```python
from build123d import *

# Parameters (mm, degrees)
F1_DEPTH  = 27
F2_R      = 4
F3_DEPTH  = 2
F4_DEPTH  = 29
F5_R      = 9.5
F6_DEPTH  = 4.5
F7_DEPTH  = 31.5
F8_R      = 4
F9_DEPTH  = 1
F11_DEPTH = 15
F12_R     = 4
F13_DEPTH = 0.1
F14_R     = 18.5
F15_DEPTH = 58
F16_R     = 2
F17_DEPTH = 1.5
F18_R     = 1.49999
F19_R     = 2
F20_DEPTH = 5
F21_R     = 2
F22_DEPTH = 5


# Not quite as in the source:
# - a fillet or chamfer is up to 0.001 mm smaller than in the source, because OpenCascade refuses the exact size


with BuildPart() as f1:
    # F0 (on Top) → F1 (new body)
    with BuildSketch(Plane.XY):
        with BuildLine():
            ThreePointArc((38, 17), (37.1213203436, 19.1213203436), (35, 20))
            Line((35, 20), (-17, 20))
            ThreePointArc((-17, 20), (-19.1213203436, 19.1213203436), (-20, 17))
            Line((-20, 17), (-20, -17))
            ThreePointArc((-20, -17), (-19.1213203436, -19.1213203436), (-17, -20))
            Line((-17, -20), (35, -20))
            ThreePointArc((35, -20), (37.1213203436, -19.1213203436), (38, -17))
            Line((38, -17), (38, 17))
        make_face()
    extrude(amount=F1_DEPTH)

    # F2 (on face) → F3 (join)
    with BuildSketch(Plane.XY.offset(27)):
        with Locations((-11, 14)):
            Circle(F2_R)
        with Locations((29, 14)):
            Circle(F2_R)
        with Locations((-11, -14)):
            Circle(F2_R)
        with BuildLine():
            Line((32.4641016151, -12), (29.9641016151, -7.6698729811))
            ThreePointArc((29.9641016151, -7.6698729811), (24.5, -6.2057713659), (23.0358983849, -11.6698729811))
            Line((23.0358983849, -11.6698729811), (25.5358983849, -16))
            ThreePointArc((25.5358983849, -16), (31, -17.4641016151), (32.4641016151, -12))
        make_face()
        with Locations((15.5, 6)):
            Circle(F2_R)
        with Locations((15.5, -6)):
            Circle(F2_R)
    extrude(amount=F3_DEPTH)

    # F2 (on face) → F4 (join)
    with BuildSketch(Plane.XY.offset(27)):
        with Locations((-11, 14)):
            Circle(F2_R)
        with Locations((29, 14)):
            Circle(F2_R)
        with Locations((-11, -14)):
            Circle(F2_R)
        with BuildLine():
            Line((32.4641016151, -12), (29.9641016151, -7.6698729811))
            ThreePointArc((29.9641016151, -7.6698729811), (24.5, -6.2057713659), (23.0358983849, -11.6698729811))
            Line((23.0358983849, -11.6698729811), (25.5358983849, -16))
            ThreePointArc((25.5358983849, -16), (31, -17.4641016151), (32.4641016151, -12))
        make_face()
        with Locations((15.5, 6)):
            Circle(F2_R)
        with Locations((15.5, -6)):
            Circle(F2_R)
    extrude(amount=-F4_DEPTH)

    # F5 (on face) → F6 (join)
    with BuildSketch(Plane.XY.offset(27)):
        Circle(F5_R)
    extrude(amount=F6_DEPTH)

    # F5 (on face) → F7 (join)
    with BuildSketch(Plane.XY.offset(27)):
        Circle(F5_R)
    extrude(amount=-F7_DEPTH)

    # F8 (on face) → F9 (join)
    with BuildSketch(Plane.XY.offset(31.5)):
        Circle(F8_R)
    extrude(amount=F9_DEPTH)

    # F10 (on face) → F11 (join)
    with BuildSketch(Plane.XY.offset(32.5)):
        with BuildLine():
            Line((2.6457513111, 3), (-2.6457513111, 3))
            ThreePointArc((-2.6457513111, 3), (0, -4), (2.6457513111, 3))
        make_face()
    extrude(amount=F11_DEPTH)

    # F12 (on face) → F13 (cut)
    with BuildSketch(Plane(origin=(0, 0, -4.5), x_dir=(1, 0, 0), z_dir=(0, 0, -1))):
        Circle(F12_R)
    extrude(amount=-F13_DEPTH, mode=Mode.SUBTRACT)

    # F14 (on face) → F15 (join)
    with BuildSketch(Plane.YZ.offset(38)):
        with Locations((0, 8.5)):
            Circle(F14_R)
    extrude(amount=F15_DEPTH)

    # F16 (on face) → F17 (join)
    with BuildSketch(Plane.XY.offset(27)):
        with Locations((-17, 17)):
            Circle(F16_R)
        with Locations((35, 17)):
            Circle(F16_R)
        with Locations((35, -17)):
            Circle(F16_R)
        with Locations((-17, -17)):
            Circle(F16_R)
    extrude(amount=F17_DEPTH)

    # F18 (radius 1.5 in the source; OpenCascade refuses exactly that, so slightly less here)
    f18_edges = [f1.edges().sort_by_distance(p)[0] for p in [
        (-19, 17, 28.5),
        (-19, -17, 28.5),
        (33, -17, 28.5),
        (33, 17, 28.5),
    ]]
    fillet(f18_edges, radius=F18_R)

    # F19 (on face) → F20 (cut)
    with BuildSketch(Plane.XY.offset(29)):
        with Locations((-11, 14)):
            Circle(F19_R)
        with Locations((-11, -14)):
            Circle(F19_R)
        with Locations((29, -14)):
            Circle(F19_R)
        with Locations((29, 14)):
            Circle(F19_R)
    extrude(amount=-F20_DEPTH, mode=Mode.SUBTRACT)

    # F21 (on face) → F22 (cut)
    with BuildSketch(Plane(origin=(0, 0, -2), x_dir=(1, 0, 0), z_dir=(0, 0, -1))):
        with Locations((29, 14)):
            Circle(F21_R)
        with Locations((29, -14)):
            Circle(F21_R)
        with Locations((-11, -14)):
            Circle(F21_R)
        with Locations((-11, 14)):
            Circle(F21_R)
    extrude(amount=-F22_DEPTH, mode=Mode.SUBTRACT)


solid = f1.part
```
Verification items for the finished model (mm, model axes). A direction names the side the tool comes from. Give positions to 0.01 mm unless a question says otherwise; leave off trailing zeros. Order: outer loops, then holes, each group sorted by start corner. A loop starts at its lowest first (then second) coordinate and runs counter-clockwise, first axis right, second up. Notation, with made-up numbers: (-19.75, -31.5) - (13.25, -31.5) arc R30 ccw to (13.25, 2.5) - close; hole circle Ø4 at (-22, -5). An arc over 180 degrees is marked (long way). Answer as CSV lines item,"result". Start each with the question number.
Item 1: Access from +Z, -Z, +X, -X, +Y, -Y to the whole of each face (thin tool, end or side, straight path). Record for faces 3 (the face through (29, -14, 24)), 4 (the face through (0, 3, 40)), 5 (the face through (12.3, 3.6, -1)).
Item 2: Gauge pin test, flat ends, axial feed: pin 1 (9 mm diameter, centred on x = -1, y = -1, fed in from -Z); pin 2 (3 mm diameter, centred on x = -11, y = -14, fed in from -Z); pin 3 (0.8 mm diameter, centred on x = 35, y = -17, fed in from +Z). Record the tip position at first contact, or that the pin passes through.
Item 3: Section check D-D, the plane x = 0.5. Record the boundary of the cut face in (y, z), plus the area to 3 significant figures.
Item 4: Section check A-A, the plane z = 8.5. Record the boundary of the cut face in (x, y), plus the area to 3 significant figures.
Item 5: Section check B-B, the plane y = 6. Record the boundary of the cut face in (x, z).
Item 6: Section check C-C, the plane x = 61.5. Record the boundary of the cut face in (y, z).
Item 7: Material ranges on L1, parallel to X at y = 14, z = 0.9; L2, parallel to Z at x = 19, y = -8.5; L3, parallel to Z at x = 48, y = -17, recorded low to high.
Item 8: Mould release check, pull along X, two halves, no side actions. Record for faces 1 (the face through (29, 14, 3)), 2 (the face through (28, -12, 29)): released by +X, released by -X, zero draft, split by the parting line, or undercut.
Filled in:
1,face 3,"+Z"
1,face 4,"+Z, +X, -X, +Y"
1,face 5,"-Z"
2,pin 1,"z = -4.5"
2,pin 2,"z = 3"
2,pin 3,"z = 28.5"
3,outline,"(-20, 0) - (-9.49, 0) - (-9.49, -4.5) - (-3.97, -4.5) - (-3.97, -4.4) - (3.97, -4.4) - (3.97, -4.5) - (9.49, -4.5) - (9.49, 0) - (20, 0) - (20, 27) - (9.49, 27) - (9.49, 31.5) - (3.97, 31.5) - (3.97, 32.5) - (3, 32.5) - (3, 47.5) - (-3.97, 47.5) - (-3.97, 31.5) - (-9.49, 31.5) - (-9.49, 27) - (-20, 27) - close"
3,area,"1,360 mm^2"
4,outline,"(-20, -17) arc R3 ccw to (-17, -20) - (35, -20) arc R3 ccw to (38, -17) - (38, -18.5) - (96, -18.5) - (96, 18.5) - (38, 18.5) - (38, 17) arc R3 ccw to (35, 20) - (-17, 20) arc R3 ccw to (-20, 17) - close"
4,area,"4,460 mm^2"
5,outline,"(-20, 0) - (-7.37, 0) - (-7.37, -4.5) - (7.37, -4.5) - (7.37, 0) - (11.5, 0) - (11.5, -2) - (19.5, -2) - (19.5, 0) - (38, 0) - (38, -9) - (96, -9) - (96, 26) - (38, 26) - (38, 27) - (19.5, 27) - (19.5, 29) - (11.5, 29) - (11.5, 27) - (7.37, 27) - (7.37, 31.5) - (-7.37, 31.5) - (-7.37, 27) - (-20, 27) - close"
6,outline,"circle Ø37 at (0, 8.5)"
7,L1,"-20 to -13, -9 to 27, 31 to 96"
7,L2,"0 to 27"
7,L3,"1.2 to 15.8"
8,face 1,"undercut"
8,face 2,"zero draft"
